```python
from build123d import *

# Parameters (mm, degrees)
F0_R      = 10
F1_DEPTH  = 20
F2_R      = 10
F3_DEPTH  = 50
F4_R      = 1.55
F5_DEPTH  = 2.6
F5_FACE_R = 1.55
F6_DEPTH  = 8


with BuildPart() as f1:
    # F0 (on Top) → F1 (new body)
    with BuildSketch(Plane.XY):
        Circle(F0_R)
    extrude(amount=F1_DEPTH)

    # F2 (on Right) → F3 (cut, symmetric)
    with BuildSketch(Plane.YZ):
        with Locations((18, 10)):
            Circle(F2_R)
        with Locations((-18, 10)):
            Circle(F2_R)
    extrude(amount=F3_DEPTH, both=True, mode=Mode.SUBTRACT)

    # F4 (on face) → F5 (cut)
    with BuildSketch(Plane(origin=(0, 0, 0), x_dir=(1, 0, 0), z_dir=(0, 0, -1))):
        Polygon((1.645448, 2.85), (-1.645448, 2.85), (-3.290897, 0), (-1.645448, -2.85), (1.645448, -2.85), (3.290897, 0), align=None)
        Circle(F4_R, mode=Mode.SUBTRACT)
    extrude(amount=-F5_DEPTH, mode=Mode.SUBTRACT)

    # F5_face (on face) → F6 (cut)
    with BuildSketch(Plane(origin=(0, 0, 0), x_dir=(1, 0, 0), z_dir=(0, 0, -1))):
        Circle(F5_FACE_R)
    extrude(amount=-F6_DEPTH, mode=Mode.SUBTRACT)


solid = f1.part
```
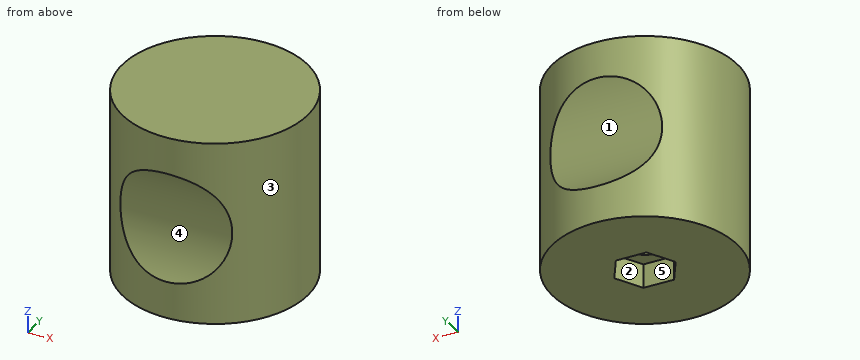
Check sheet for the modelled part. Datum: model origin and axes. Units: mm. Face numbers are marked on the shaded views. A direction names the side the tool comes from. Coordinates: 2 decimals unless noted, no trailing zeros. Write each loop counter-clockwise with the first axis right and the second up, starting at its lowest first coordinate (ties: lowest second). Pieces come first, ordered by that corner, then holes. Notation, with made-up numbers: (-28, 58.25) -> (15, 58.25) arc R19 cw to (15, 73.25) -> close; hole circle Ø4 at (74, 59.5). An arc over 180 degrees is marked (long way). Use a Markdown table: item, result.
1. Sectioned sample at A-A (x = 0). Enter the section's corners in (y, z), plus the area to 3 significant figures.
Reported:
| item | result |
|---|---|
| outline | (-10, 0) -> (-2.85, 0) -> (-2.85, 2.6) -> (-1.55, 2.6) -> (-1.55, 8) -> (1.55, 8) -> (1.55, 2.6) -> (2.85, 2.6) -> (2.85, 0) -> (10, 0) -> (10, 4) arc R10 cw to (10, 16) -> (10, 20) -> (-10, 20) -> (-10, 16) arc R10 cw to (-10, 4) -> close |
| area | 336 mm2 |
2. Go/stop test with flat-tipped pins: pin 1 Ø2.5 at (x, y) = (0.5, -0.5) entering from -Z; pin 2 Ø3 at (x, z) = (-4.5, 5.5) entering from -Y; pin 3 Ø6 at (y, z) = (-4.5, 15) entering from -X. Record where each tip stops, or that it passes through.
Reported:
| item | result |
|---|---|
| pin 1 | stops at z = 2.6 |
| pin 2 | stops at y = -9.48 |
| pin 3 | stops at x = -9.89 |
3. Sectioned sample at C-C (z = 6.5). Enter the section's corners in (x, y), plus the area to 3 significant figures.
Reported:
| item | result |
|---|---|
| outline | (-5.05, -8.63) -> (5.05, -8.63) arc R10 ccw to (5.05, 8.63) -> (-5.05, 8.63) arc R10 ccw to start; hole circle Ø3.1 at (0, 0) |
| area | 288 mm2 |
4. Sectioned sample at B-B (y = -2.25). Enter the section's corners in (x, z), plus the area to 3 significant figures.
Reported:
| item | result |
|---|---|
| outline | (-9.74, 0) -> (-1.99, 0) -> (-1.99, 2.6) -> (1.99, 2.6) -> (1.99, 0) -> (9.74, 0) -> (9.74, 20) -> (-9.74, 20) -> close |
| area | 379 mm2 |
5. Tool access check on the marked faces 4 and 5. Record the directions out of +Z, -Z, +X, -X, +Y, -Y that give a thin tool (end or side, any length) a straight path to the whole face; none if there is none.
Reported:
| item | result |
|---|---|
| face 4 | +X, -X, -Y |
| face 5 | -Z |
6. Release check for a two-part mould opening along Y. For the marked faces 1, 2 and 3 record: pulls with the +Y half, pulls with the -Y half, needs draft (parallel to the pull), parting line crosses it, or undercut.
Reported:
| item | result |
|---|---|
| face 1 | pulls with the +Y half |
| face 2 | undercut |
| face 3 | parting line crosses it |
7. Sectioned sample at D-D (x = -3). Enter the section's corners in (y, z).
Reported:
| item | result |
|---|---|
| outline | (-9.54, 0) -> (-0.5, 0) -> (-0.5, 2.6) -> (0.5, 2.6) -> (0.5, 0) -> (9.54, 0) -> (9.54, 4.67) arc R10 cw to (9.54, 15.33) -> (9.54, 20) -> (-9.54, 20) -> (-9.54, 15.33) arc R10 cw to (-9.54, 4.67) -> close |
8. Scan lines: line 1 along Y through (x, z) = (0, 3.9); line 2 along Y through (x, z) = (6, 9.5); line 3 along Z through (x, y) = (1.5, -0.75). Record each from-to range of solid material in increasing order.
Reported:
| item | result |
|---|---|
| line 1 | y = -10 to -1.55, 1.55 to 10 |
| line 2 | y = -8 to 8 |
| line 3 | z = 2.6 to 20 |
